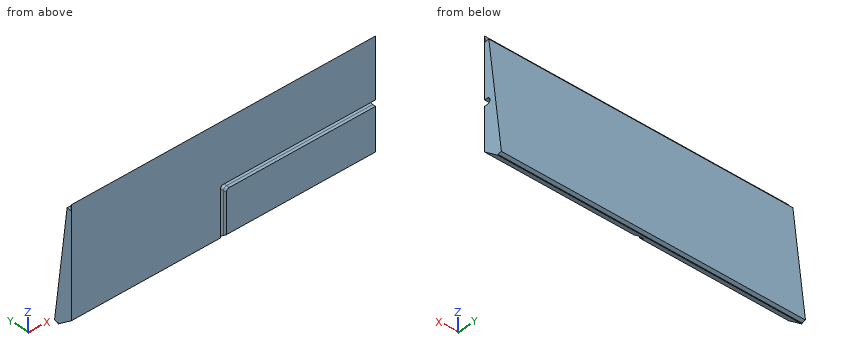
from build123d import *

# Parameters (mm, degrees)
SKETCH2_W           = 121.3
SKETCH2_H           = 304.5
BOSS_EXTRUDE1_DEPTH = 20
CUT_EXTRUDE2_DEPTH  = 329.94119958
SKETCH6_W           = 6
SKETCH6_H           = 6
CUT_EXTRUDE3_DEPTH  = 155.4
SKETCH8_W           = 6
SKETCH8_H           = 6
CUT_EXTRUDE4_DEPTH  = 312.915359451
FILLET2_R           = 3


with BuildPart() as part:
    # Sketch2 → Boss-Extrude1 (new body)
    with BuildSketch(Plane(origin=(0, 0, 0), x_dir=(0, 0.12186934340514809, -0.992546151641322), z_dir=(0, -0.992546151641322, -0.12186934340514809))):
        with Locations((60.65, 152.25)):
            Rectangle(SKETCH2_W, SKETCH2_H)
    extrude(amount=BOSS_EXTRUDE1_DEPTH)

    # Sketch4 → Cut-Extrude2 (cut, through all)
    with BuildSketch(Plane(origin=(304.5, 0, 0), x_dir=(0, 0, -1), z_dir=(1, 0, 0))):
        Polygon((109.333774414, -3.970184607), (0.487477374, -3.970184607), (2.437386868, -19.850923033), (122.833235062, -5.068171678), (120.883325568, 10.812566748), align=None)
        Polygon((5.95527691, 0.73121606), (0, 0), (0.487477374, -3.970184607), (6.442754283, -3.238968546), align=None)
        Polygon((120.883325568, 10.812566748), (120.395848194, 14.782751355), (119.403302042, 14.660882012), (119.890779416, 10.690697405), align=None)
    extrude(amount=-CUT_EXTRUDE2_DEPTH, mode=Mode.SUBTRACT)

    # Sketch6 → Cut-Extrude3 (cut)
    with BuildSketch(Plane(origin=(304.5, 0, 0), x_dir=(0, 0, -1), z_dir=(1, 0, 0))):
        with Locations((63.487477374, -0.970184607)):
            Rectangle(SKETCH6_W, SKETCH6_H)
    extrude(amount=-CUT_EXTRUDE3_DEPTH, mode=Mode.SUBTRACT)

    # Sketch8 → Cut-Extrude4 (cut, through all)
    with BuildSketch(Plane.XY.offset(-66.487477374)):
        with Locations((152.1, -0.970184607)):
            Rectangle(SKETCH8_W, SKETCH8_H)
    extrude(amount=-CUT_EXTRUDE4_DEPTH, mode=Mode.SUBTRACT)

    # Fillet2
    fillet2_edges = [part.edges().sort_by_distance(p)[0] for p in [
        (155.1, 2.029815393, -90.254482773),
        (149.1, 2.029815393, -87.254482773),
        (229.8, 2.029815393, -66.487477374),
        (226.8, 2.029815393, -60.487477374),
        (155.1, -0.970184607, -66.487477374),
        (149.1, -0.970184607, -60.487477374),
    ]]
    fillet(fillet2_edges, radius=FILLET2_R - 0.0001)  # a hair under: the kernel refuses the full size


solid = part.part
Geometry check sheet. Reference: the model listing, model coordinates, mm. Give positions to 0.01 mm unless a question says otherwise; leave off trailing zeros. Write each loop counter-clockwise with the first axis right and the second up, starting at its lowest first coordinate (ties: lowest second). Pieces come first, ordered by that corner, then holes. Notation, with made-up numbers: M 76.5,36.5 L 108.5,36.5 A23 cw 108.5,60.5 Z; hole C 21.5,15.25 d5. An arc over 180 degrees is marked long. One line per question, with ' | ' between items.
1. Cross-section at D-D (y = 6.25). Enter the section's corners in (x, z).
Ans:
outline: M 0,-117.32 L 304.5,-117.32 L 304.5,-50.9 L 0,-50.9 Z
2. Cross-section at A-A (x = 68.5). Enter the section's corners in (y, z), plus the area to 3 significant figures.
Ans:
outline: M -3.97,-109.33 L 10.81,-120.88 L 10.69,-119.89 L 14.66,-119.4 L 0.73,-5.96 L -3.24,-6.44 L -3.97,-0.49 Z | area: 1,260 mm2
3. Scan lines: line 1 along X through (y, z) = (-1.75, -92.5); line 2 along Z through (x, y) = (289.5, -3); line 3 along Z through (x, y) = (239.5, 0). Record each from-to range of solid material in increasing order. Write a range as from..to.
Ans:
line 1: 0..149.1, 155.1..304.5 | line 2: -110.09..-66.49, -60.49..-6.41 | line 3: -112.44..-66.33, -60.65..-6.05
4. Gauge pin test, flat ends, axial feed: pin 1 (5 mm diameter, centred on x = 216, z = -66, fed in from -Y); pin 2 (1.5 mm diameter, centred on x = 263.5, y = -2.5, fed in from -Z); pin 3 (8 mm diameter, centred on x = 136.5, y = 4.5, fed in from -Z); pin 4 (0.9 mm diameter, centred on x = 213, y = -2, fed in from +Z). Record the tip position at first contact, or that the pin passes through.
Ans:
pin 1: y = -3.97 | pin 2: z = -111.07 | pin 3: z = -119.08 | pin 4: z = -6.24
